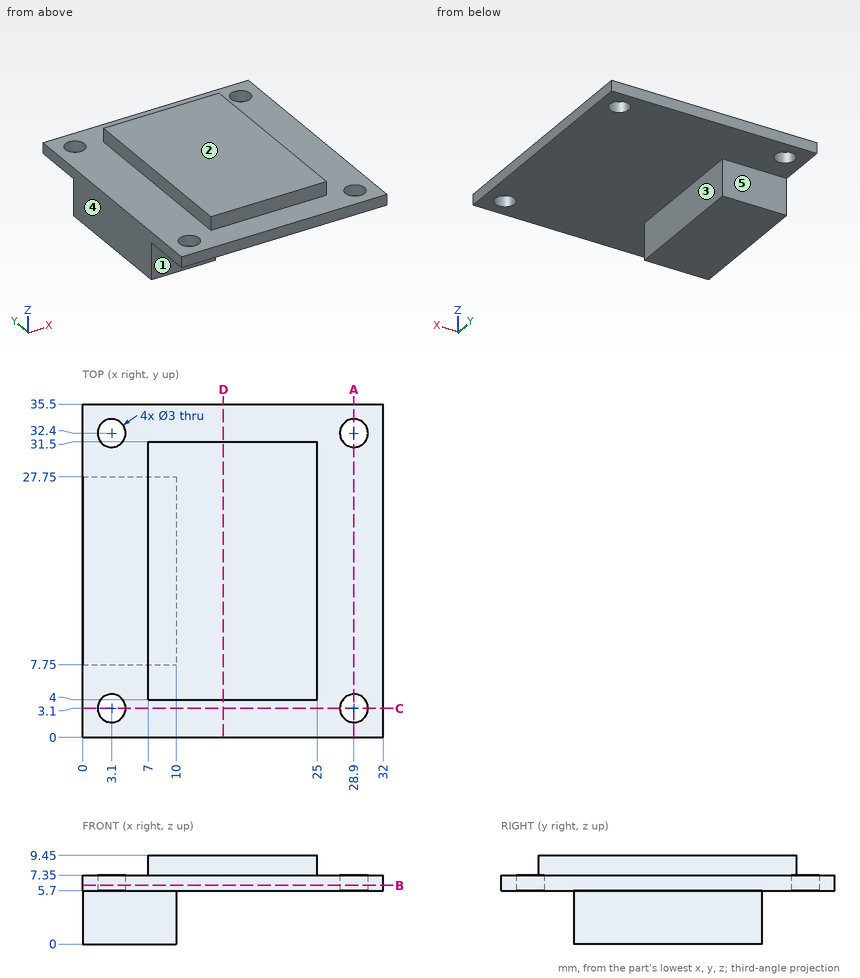
Study the drawing (mm; zero at the part's minimum x, y, z) and answer. A direction names the side the tool comes from. Coordinates: 2 decimals unless noted, no trailing zeros. Write each loop counter-clockwise with the first axis right and the second up, starting at its lowest first coordinate (ties: lowest second). Pieces come first, ordered by that corner, then holes.
Q1. Which of the six approach directions +Z, -Z, +X, -X, +Y, -Y give full straight-line access (tool end or side, diameter ignored) to the marked faces 1, 2, 3, 4 and 5?
Q2. A cutting plane is placed at D-D, the plane x = 15. Give the vertices of the cut face in (y, z).
Q3. A cutting plane is placed at B-B, the plane z = 6.25. Give the vertices of the cut face in (x, y).
Q4. Each of these flat-tipped pins is pushed along its axis until it touches: pin 1 Ø1.7 at (x, z) = (3, 4.5) entering from -Y; pin 2 Ø1.7 at (x, z) = (19, 8.5) entering from +Y; pin 3 Ø4 at (x, y) = (3.1, 32.4) entering from +Z. Where does it stop, or does it pass through?
Q5. A cutting plane is placed at C-C, the plane y = 3.1. Give the vertices of the cut face in (x, z), then the cut area to 3 significant figures.
Q6. Find the intervals of material crossed by line 1 (Y direction, x = 3.1, z = 6.45); line 2 (X direction, y = 11.5, z = 1); line 3 (Z direction, x = 14, y = 12), in increasing order.
Q7. A cutting plane is placed at A-A, the plane x = 28.9. Give the vertices of the cut face in (y, z), then the cut area to 3 significant figures.
Findings below:
1. face 1: -Z, +X, -X, -Y
1. face 2: +Z, +X, -X, +Y, -Y
1. face 3: -Z, +X, +Y, -Y
1. face 4: +Z, -Z, -X, +Y, -Y
1. face 5: -Z, +X, -X, +Y
2. outline: (0, 5.7) - (35.5, 5.7) - (35.5, 7.35) - (31.5, 7.35) - (31.5, 9.45) - (4, 9.45) - (4, 7.35) - (0, 7.35) - close
3. outline: (0, 0) - (32, 0) - (32, 35.5) - (0, 35.5) - close; hole circle Ø3 at (3.1, 3.1); hole circle Ø3 at (3.1, 32.4); hole circle Ø3 at (28.9, 3.1); hole circle Ø3 at (28.9, 32.4)
4. pin 1: stops at y = 7.75
4. pin 2: stops at y = 31.5
4. pin 3: stops at z = 7.35
5. outline: (0, 5.7) - (1.6, 5.7) - (1.6, 7.35) - (0, 7.35) - close; (4.6, 5.7) - (27.4, 5.7) - (27.4, 7.35) - (4.6, 7.35) - close; (30.4, 5.7) - (32, 5.7) - (32, 7.35) - (30.4, 7.35) - close
5. area: 42.9 mm2
6. line 1: y = 0 to 1.6, 4.6 to 30.9, 33.9 to 35.5
6. line 2: x = 0 to 10
6. line 3: z = 5.7 to 9.45
7. outline: (0, 5.7) - (1.6, 5.7) - (1.6, 7.35) - (0, 7.35) - close; (4.6, 5.7) - (30.9, 5.7) - (30.9, 7.35) - (4.6, 7.35) - close; (33.9, 5.7) - (35.5, 5.7) - (35.5, 7.35) - (33.9, 7.35) - close
7. area: 48.7 mm2
